The model under review builds one solid part; all positions refer to its coordinate system, in mm. Face numbers are marked on the shaded views. A direction names the side the tool comes from. Round coordinates to 2 decimals unless told otherwise and drop trailing zeros. Use one line per item in the form item = value.
from build123d import *

# Parameters (mm, degrees)
F0_R           = 38.5
F1_DEPTH       = 6.9
F0_R_2         = 51.5
F2_DEPTH       = 5
F4_D           = 6.6
F4_CBORE_D     = 11.25
F4_CBORE_DEPTH = 6
F6_D           = 5.5
F6_DEPTH       = 9
F6_TIP         = 1.6523667023
F7_R           = 4.99999
F8_SIZE        = 1


# Not quite as in the source:
# - a fillet or chamfer is up to 0.001 mm smaller than in the source, because OpenCascade refuses the exact size


with BuildPart() as f1:
    # F0 (on Top) → F1 (new body)
    with BuildSketch(Plane.XY):
        Circle(F0_R)
    extrude(amount=-F1_DEPTH)

    # F0 (on Top) → F2 (join)
    with BuildSketch(Plane.XY):
        Circle(F0_R_2)
        Circle(F0_R, mode=Mode.SUBTRACT)
        Circle(F0_R)
    extrude(amount=F2_DEPTH)

    # F4 (through all)
    with Locations(Plane(origin=(0, 0, -6.9), x_dir=(1, 0, 0), z_dir=(0, 0, -1))):
        with Locations((-15.1554445662, -8.75), (0, 17.5), (15.1554445662, -8.75)):
            CounterBoreHole(F4_D / 2, F4_CBORE_D / 2, F4_CBORE_DEPTH)

    # F6
    with Locations(Plane(origin=(0, 0, -6.9), x_dir=(1, 0, 0), z_dir=(0, 0, -1))):
        with Locations((-12, 0), (12, 0)):
            Hole(F6_D / 2, depth=F6_DEPTH)
            with Locations((0, 0, -(F6_DEPTH + F6_TIP / 2))):  # 118° drill point
                Cone(0, F6_D / 2, F6_TIP, mode=Mode.SUBTRACT)

    # F7 (radius 5 in the source; OpenCascade refuses exactly that, so slightly less here)
    f7_edges = [f1.edges().sort_by_distance(p)[0] for p in [
        (-51.5, 0, 5),
    ]]
    fillet(f7_edges, radius=F7_R)

    # F8
    f8_edges = [f1.edges().sort_by_distance(p)[0] for p in [
        (-38.5, 0, -6.9),
    ]]
    chamfer(f8_edges, length=F8_SIZE)


solid = f1.part
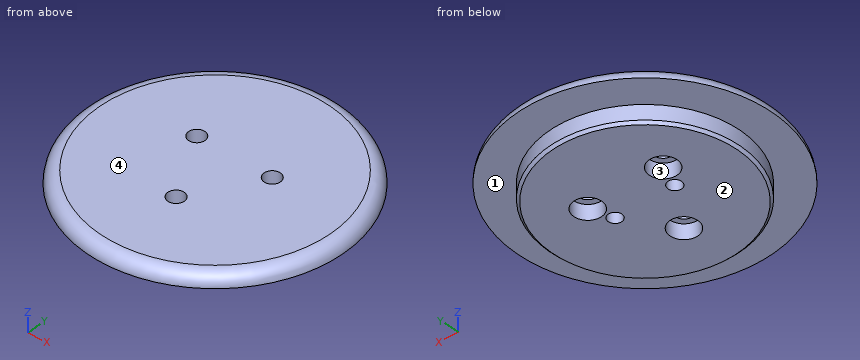
(1) Insertion check: P1, Ø3, axis at y = 25.5, z = 2, coming from the -X side; P2, Ø3.5, axis at x = 17, y = 10, coming from the -Z side; P3, Ø3, axis at x = 27.5, y = -38, coming from the -Z side. Each pin has a flat end and moves straight along its axis. Give the tip position at first contact, or say it passes through.
Geometry results:
P1 = -45.28
P2 = -0.9
P3 = 0
(2) To check wall thickness, follow L1, parallel to X at y = 8.75, z = 1.25; L2, parallel to Y at x = 9.5, z = -3.5; L3, parallel to X at y = -17.5, z = 1.85. State the ranges of each line that lie inside material, in increasing order.
Geometry results:
L1 = -50.59 to -18.46, -11.86 to 11.86, 18.46 to 50.59
L2 = -37.31 to -1.15, 1.15 to 37.31
L3 = -48.06 to -3.3, 3.3 to 48.06
(3) Machinability: for the marked faces 1 and 2, which of the approach directions +Z, -Z, +X, -X, +Y, -Y give a long, thin tool a straight path to every point of the face, cutting with its end or side? Answer none if there is none.
Geometry results:
face_1 = -Z
face_2 = -Z, +X, -X, +Y, -Y
(4) The part is to be moulded in two halves that separate along X. For the marked faces 3 and 4, say which applies: +X half, -X half, draft (parallel to the pull), parting line (faces both ways), or undercut.
Geometry results:
face_3 = undercut
face_4 = draft
(5) Add section B-B on y = 8.75. Count the separate pieces of the cut face and the enclosed holes in it, then the cut area to 3 significant figures.
Geometry results:
separate_pieces = 3
enclosed_holes = 0
area = 800 mm2
